Part model, mm, in its own coordinate system. Round coordinates to 2 decimals unless told otherwise and drop trailing zeros. Write each loop counter-clockwise with the first axis right and the second up, starting at its lowest first coordinate (ties: lowest second). Pieces come first, ordered by that corner, then holes. Notation, with made-up numbers: (84, 61.25) -> (130, 61.25) arc R32 ccw to (130, 100.25) -> close; hole circle Ø7 at (19, -31). An arc over 180 degrees is marked (long way). Return JSON: item names as keys, results as strings. Group by question number.
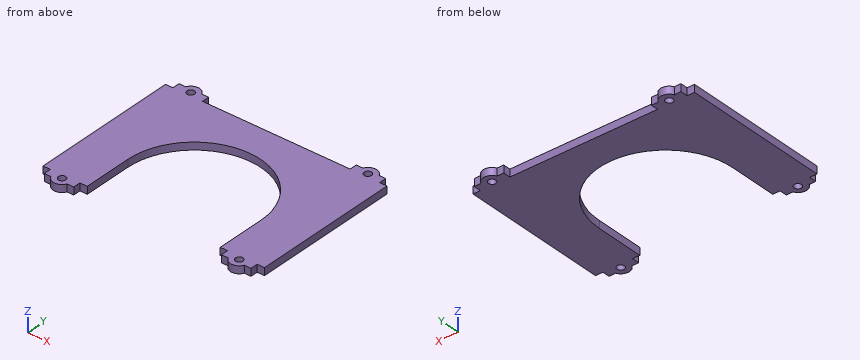
```python
from build123d import *

# Parameters (mm, degrees)
SKETCH1_W                                  = 150
SKETCH1_H                                  = 100
BOSS_EXTRUDE1_DEPTH                        = 5
SKETCH3_W                                  = 20
SKETCH3_H                                  = 5
BOSS_EXTRUDE2_DEPTH                        = 5
MIRROR1_AT_THE_SECOND_PLANE_COPY_1_SKETC_W = 20
MIRROR1_AT_THE_SECOND_PLANE_COPY_1_SKETC_H = 5
MIRROR1_AT_THE_SECOND_PLANE_COPY_1_DEPTH   = 5
SKETCH4_R                                  = 6
BOSS_EXTRUDE3_DEPTH                        = 5
SKETCH5_R                                  = 2.5
CUT_EXTRUDE1_DEPTH                         = 5
MIRROR2_AT_THE_SECOND_PLANE_COPY_1_SKETC_R = 6
MIRROR2_AT_THE_SECOND_PLANE_COPY_1_DEPTH   = 5
MIRROR2_AT_THE_SECOND_PLANE_COPY_2_SKETC_R = 2.5
MIRROR2_AT_THE_SECOND_PLANE_COPY_2_DEPTH   = 5
CUT_EXTRUDE3_DEPTH                         = 1
CUT_EXTRUDE3_DEPTH_BACK                    = 5


with BuildPart() as part:
    # Sketch1 → Boss-Extrude1 (new body)
    with BuildSketch(Plane.XY):
        Rectangle(SKETCH1_W, SKETCH1_H)
    extrude(amount=BOSS_EXTRUDE1_DEPTH)

    # Sketch3 → Boss-Extrude2 (add)
    with BuildSketch(Plane.XZ.offset(50)):
        with Locations((-60, 2.5)):
            Rectangle(SKETCH3_W, SKETCH3_H)
    boss_extrude2 = extrude(amount=BOSS_EXTRUDE2_DEPTH)

    # Mirror1: Boss-Extrude2 across plane
    add(boss_extrude2.mirror(Plane(origin=(0, 0, 0), x_dir=(0, 0, 1), z_dir=(1, 0, 0))))

    # Mirror1 at the second plane: Boss-Extrude2 across plane
    add(boss_extrude2.mirror(Plane.ZX))

    # Mirror1 at the second plane copy 1 sketc → Mirror1 at the second plane copy 1 (add)
    with BuildSketch(Plane(origin=(0, 50, 0), x_dir=(-1, 0, 0), z_dir=(0, 1, 0))):
        with Locations((-60, 2.5)):
            Rectangle(MIRROR1_AT_THE_SECOND_PLANE_COPY_1_SKETC_W, MIRROR1_AT_THE_SECOND_PLANE_COPY_1_SKETC_H)
    extrude(amount=MIRROR1_AT_THE_SECOND_PLANE_COPY_1_DEPTH)

    # Sketch4 → Boss-Extrude3 (add)
    with BuildSketch(Plane.XY.offset(5)):
        with Locations((60, 52.5)):
            Circle(SKETCH4_R)
    boss_extrude3 = extrude(amount=-BOSS_EXTRUDE3_DEPTH)

    # Sketch5 → Cut-Extrude1 (cut)
    with BuildSketch(Plane.XY.offset(5)):
        with Locations((60, 52.5)):
            Circle(SKETCH5_R)
    cut_extrude1 = extrude(amount=-CUT_EXTRUDE1_DEPTH, mode=Mode.SUBTRACT)

    # Mirror2: Boss-Extrude3, Cut-Extrude1 across plane
    add(boss_extrude3.mirror(Plane(origin=(0, 0, 0), x_dir=(0, 0, 1), z_dir=(1, 0, 0))))
    add(cut_extrude1.mirror(Plane(origin=(0, 0, 0), x_dir=(0, 0, 1), z_dir=(1, 0, 0))), mode=Mode.SUBTRACT)

    # Mirror2 at the second plane: Boss-Extrude3, Cut-Extrude1 across plane
    add(boss_extrude3.mirror(Plane.ZX))
    add(cut_extrude1.mirror(Plane.ZX), mode=Mode.SUBTRACT)

    # Mirror2 at the second plane copy 1 sketc → Mirror2 at the second plane copy 1 (add)
    with BuildSketch(Plane(origin=(0, 0, 5), x_dir=(-1, 0, 0), z_dir=(0, 0, 1))):
        with Locations((60, 52.5)):
            Circle(MIRROR2_AT_THE_SECOND_PLANE_COPY_1_SKETC_R)
    extrude(amount=-MIRROR2_AT_THE_SECOND_PLANE_COPY_1_DEPTH)

    # Mirror2 at the second plane copy 2 sketc → Mirror2 at the second plane copy 2 (cut)
    with BuildSketch(Plane(origin=(0, 0, 5), x_dir=(-1, 0, 0), z_dir=(0, 0, 1))):
        with Locations((60, 52.5)):
            Circle(MIRROR2_AT_THE_SECOND_PLANE_COPY_2_SKETC_R)
    extrude(amount=-MIRROR2_AT_THE_SECOND_PLANE_COPY_2_DEPTH, mode=Mode.SUBTRACT)

    # Sketch8 → Cut-Extrude3 (cut, two sides)
    with BuildSketch(Plane.XY.offset(5)) as cut_extrude3_sk:
        with BuildLine():
            Line((45, -383.556795633), (45, -50))
            Line((45, -50), (45, -16.928023383))
            ThreePointArc((45, -16.928023383), (0, 28.071976617), (-45, -16.928023383))
            Line((-45, -16.928023383), (-45, -50))
            Line((-45, -50), (-45, -383.556795633))
            Line((-45, -383.556795633), (-45, -1050.670386898))
            Line((-45, -1050.670386898), (45, -1050.670386898))
            Line((45, -1050.670386898), (45, -383.556795633))
        make_face()
    extrude(amount=CUT_EXTRUDE3_DEPTH, mode=Mode.SUBTRACT)
    extrude(cut_extrude3_sk.sketch, amount=-CUT_EXTRUDE3_DEPTH_BACK, mode=Mode.SUBTRACT)


solid = part.part
```
Item 1: Cut at C-C (y = -52.5). Write the cut outline in (x, z), then the cut area to 3 significant figures.
Item 2: Cut at A-A (y = -34). Write the cut outline in (x, z).
Item 3: Wall check: L1, parallel to Y at x = 60, z = 2.9; L2, parallel to X at y = -52.5, z = 2.1; L3, parallel to X at y = -41, z = 1.4. Give the ranges that are in metal, low to high.
Item 4: Flat gauge pins, fed straight in: P1, Ø1.5, axis at x = -73.5, z = 3, coming from the +Y side; P2, Ø3, axis at x = -60, y = -52.5, coming from the -Z side; P3, Ø2.5, axis at x = -68.5, z = 2.5, coming from the -Y side; P4, Ø1.5, axis at y = -51.5, z = 2.5, coming from the -X side. Where does each tip first touch, or does it go through?
Item 5: Cut at D-D (z = 1.7). State how many separate pieces and enclosed holes the cut face has, then the cut area to 3 significant figures.
Item 6: Cut at B-B (x = -60). Write the cut outline in (y, z), then the cut area to 3 significant figures.
Checks:
{
 "1": {"outline": "(-70, 0) -> (-62.5, 0) -> (-62.5, 5) -> (-70, 5) -> close; (-57.5, 0) -> (-50, 0) -> (-50, 5) -> (-57.5, 5) -> close; (50, 0) -> (57.5, 0) -> (57.5, 5) -> (50, 5) -> close; (62.5, 0) -> (70, 0) -> (70, 5) -> (62.5, 5) -> close", "area": "150 mm2"},
 "2": {"outline": "(-75, 0) -> (-45, 0) -> (-45, 5) -> (-75, 5) -> close; (45, 0) -> (75, 0) -> (75, 5) -> (45, 5) -> close"},
 "3": {"L1": "y = -58.5 to -55, -50 to 50, 55 to 58.5", "L2": "x = -70 to -62.5, -57.5 to -50, 50 to 57.5, 62.5 to 70", "L3": "x = -75 to -45, 45 to 75"},
 "4": {"P1": "stops at y = 50", "P2": "passes through", "P3": "stops at y = -55", "P4": "stops at x = -70"},
 "5": {"separate pieces": "1", "enclosed holes": "4", "area": "9,270 mm2"},
 "6": {"outline": "(-58.5, 0) -> (-55, 0) -> (-55, 5) -> (-58.5, 5) -> close; (-50, 0) -> (50, 0) -> (50, 5) -> (-50, 5) -> close; (55, 0) -> (58.5, 0) -> (58.5, 5) -> (55, 5) -> close", "area": "535 mm2"}
}
